from build123d import *

# Parameters (mm, degrees)
F0_W     = 2.8575
F0_H     = 5.08
F0_W_2   = 1.905
F0_W_3   = 5.3975
F0_H_2   = 5.128411484
F1_DEPTH = 4.445
F2_W     = 7.62
F2_H     = 83.82
F3_DEPTH = 5.3975
F4_W     = 17.018
F4_H     = 2.54
F4_W_2   = 2.45618
F4_W_3   = 14.56182
F5_DEPTH = 15.24
F6_DEPTH = 25.4


# Not quite as in the source:
# - a feature names something its author has since deleted; it is built from what else it names


with BuildPart() as f1:
    # F0 (on Front) → F1 (new body, symmetric)
    with BuildSketch(Plane.XZ):
        with Locations((-63.4578398415, 18.0266693214)):
            Rectangle(F0_W, F0_H)
        Polygon((-62.0290898415, 15.4866693214), (-64.8865898415, 15.4866693214), (-64.8865898415, 5.3266693214), (-1.3865898415, 5.3266693214), (-1.3865898415, 15.4866693214), (-6.7840898415, 15.4866693214), (-8.6890898415, 15.4866693214), (-10.5940898415, 15.4866693214), (-12.4990898415, 15.4866693214), (-13.314443469, 15.4866693214), (-14.4040898415, 15.4866693214), (-16.3090898415, 15.4866693214), (-18.2140898415, 15.4866693214), (-20.1190898415, 15.4866693214), (-22.0240898415, 15.4866693214), (-23.9290898415, 15.4866693214), (-25.8340898415, 15.4866693214), (-27.7390898415, 15.4866693214), (-29.6440898415, 15.4866693214), (-31.5490898415, 15.4866693214), (-33.4540898415, 15.4866693214), (-35.3590898415, 15.4866693214), (-37.2640898415, 15.4866693214), (-39.1690898415, 15.4866693214), (-41.0740898415, 15.4866693214), (-42.9790898415, 15.4866693214), (-44.8840898415, 15.4866693214), (-46.7890898415, 15.4866693214), (-48.6940898415, 15.4866693214), (-50.5990898415, 15.4866693214), (-52.5040898415, 15.4866693214), (-54.4090898415, 15.4866693214), (-56.3140898415, 15.4866693214), (-58.2190898415, 15.4866693214), (-60.1240898415, 15.4866693214), align=None)
        with Locations((-59.1715898415, 18.0266693214)):
            Rectangle(F0_W_2, F0_H)
        with Locations((-4.0853398415, 18.0266693214)):
            Rectangle(F0_W_3, F0_H)
        with Locations((-55.3615898415, 18.0266693214)):
            Rectangle(F0_W_2, F0_H)
        with Locations((-9.6415898415, 18.0266693214)):
            Rectangle(F0_W_2, F0_H)
        with Locations((-51.5515898415, 18.0266693214)):
            Rectangle(F0_W_2, F0_H)
        Polygon((-13.314443469, 15.4866693214), (-12.4990898415, 15.4866693214), (-12.4990898415, 20.5666693214), (-13.314443469, 20.5666693214), (-14.4040898415, 20.5666693214), (-14.4040898415, 15.4866693214), align=None)
        with Locations((-47.7415898415, 18.0266693214)):
            Rectangle(F0_W_2, F0_H)
        with Locations((-43.9315898415, 18.0266693214)):
            Rectangle(F0_W_2, F0_H)
        with Locations((-17.2615898415, 18.0266693214)):
            Rectangle(F0_W_2, F0_H)
        with Locations((-40.1215898415, 18.0266693214)):
            Rectangle(F0_W_2, F0_H)
        with Locations((-21.0715898415, 18.0266693214)):
            Rectangle(F0_W_2, F0_H)
        with Locations((-36.3115898415, 18.0508750634)):
            Rectangle(F0_W_2, F0_H_2)
        with Locations((-24.8815898415, 18.0266693214)):
            Rectangle(F0_W_2, F0_H)
        with Locations((-32.5015898415, 18.0266693214)):
            Rectangle(F0_W_2, F0_H)
        with Locations((-28.6915898415, 18.0266693214)):
            Rectangle(F0_W_2, F0_H)
    extrude(amount=F1_DEPTH, both=True)

    # F2 (on face) → F3 (join)
    with BuildSketch(Plane.YZ.offset(-1.3865898415)):
        Polygon((-4.445, 5.3266693214), (-4.445, 20.5666693214), (-43.815, 20.5666693214), (-43.815, 5.3266693214), (-37.465, 5.3266693214), (-29.845, 5.3266693214), align=None)
        with Locations((-33.655, -36.5833306786)):
            Rectangle(F2_W, F2_H)
    extrude(amount=-F3_DEPTH)

    # F4 (on face) → F5 (join)
    with BuildSketch(Plane.XY.offset(20.5666693214)):
        with Locations((-15.2930898415, -19.685)):
            Rectangle(F4_W, F4_H)
        with Locations((-22.5739998415, -42.545)):
            Rectangle(F4_W_2, F4_H)
        with Locations((-14.0649998415, -42.545)):
            Rectangle(F4_W_3, F4_H)
    extrude(amount=-F5_DEPTH)

    # F2 (on face) → F6 (join)
    with BuildSketch(Plane.YZ.offset(-1.3865898415)):
        Polygon((-19.840323447, -78.4933306786), (-29.845, -78.4933306786), (-37.465, -78.4933306786), (-47.469676553, -78.4933306786), (-47.469676553, -86.1133306786), (-19.840323447, -86.1133306786), align=None)
    extrude(amount=-F6_DEPTH)


solid = f1.part
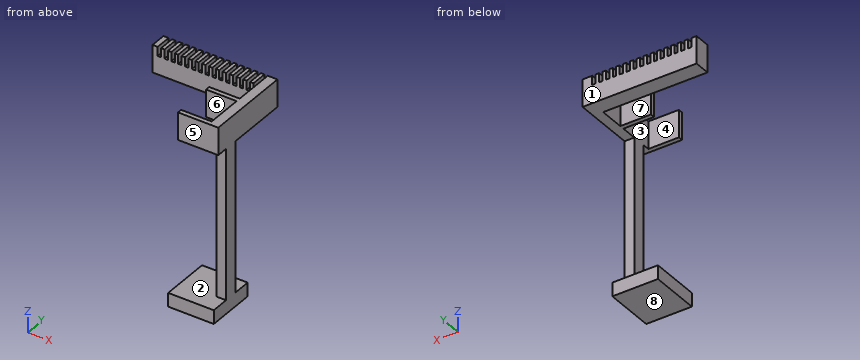
The listing builds one solid part. Answer for the finished solid, in the listing's coordinates (mm). Face numbers are marked on the shaded views. A direction names the side the tool comes from. Round coordinates to 2 decimals unless told otherwise and drop trailing zeros. Order: outer loops, then holes, each group sorted by start corner. A loop starts at its lowest first (then second) coordinate and runs counter-clockwise, first axis right, second up. Notation, with made-up numbers: (78.5, 10.25) - (103.5, 10.25) arc R33 cw to (103.5, 41.25) - close; hole circle Ø3 at (33, 73). An arc over 180 degrees is marked (long way). Write item = value, one per line. Start each with the question number.
1) Section C-C, the plane z = -23 is taken. Write down the section's boundary in (x, y) (3 decimals), plus the area to 3 significant figures.
2) Section B-B, the plane y = -6.5 is taken. Write down the section's boundary in (x, z).
3) Section A-A, the plane z = 6.5 is taken. Write down the section's boundary in (x, y) (3 decimals), plus the area to 3 significant figures.
4) For the marked faces 5, 6, 7 and 8, determine the directions among +Z, -Z, +X, -X, +Y, -Y from which every point of the face is accessible in a straight line to the end or side of a thin tool.
5) Given pin 1 (17 mm diameter, centred on x = -47.5, y = -11, fed in from -Z); pin 2 (2 mm diameter, centred on x = -23, y = -1.5, fed in from +Z); pin 3 (6.5 mm diameter, centred on x = -12, y = -29, fed in from +Z), each flat-ended and moving along its own axis, determine where each tip first touches the part or whether it passes through.
6) For a pull along Y with two mould halves and no side action, classify the marked faces 1, 2, 3 and 4 as released by +Y, released by -Y, zero draft, split by the parting line, or undercut.
7) Straight lines are drawn through the part: L1, parallel to Z at x = -14.5, y = -41.5; L2, parallel to Y at x = -45.5, z = 9 (3 decimals); L3, parallel to X at y = -31.5, z = -2. For each, find the intervals that lie inside material, in ascending order.
Results list:
q1.outline = (-6.784, -37.465) - (-1.387, -37.465) - (-1.387, -29.845) - (-6.784, -29.845) - close
q1.area = 41.1 mm^2
q2.outline = (-6.78, 5.33) - (-1.39, 5.33) - (-1.39, 20.57) - (-6.78, 20.57) - close
q3.outline = (-64.887, -4.445) - (-6.784, -4.445) - (-6.784, -18.415) - (-23.802, -18.415) - (-23.802, -20.955) - (-6.784, -20.955) - (-6.784, -41.275) - (-23.802, -41.275) - (-23.802, -43.815) - (-1.387, -43.815) - (-1.387, 4.445) - (-64.887, 4.445) - close
q3.area = 863 mm^2
q4.face_5 = +Z, +X, -X, -Y
q4.face_6 = +Z, -X
q4.face_7 = +Z, -Z, -X
q4.face_8 = -Z, +X, -X, +Y, -Y
q5.pin_1 = 5.33
q5.pin_2 = 20.57
q5.pin_3 = -78.49
q6.face_1 = released by +Y
q6.face_2 = zero draft
q6.face_3 = undercut
q6.face_4 = undercut
q7.L1 = -86.11 to -78.49, 5.33 to 20.57
q7.L2 = -4.445 to 4.445
q7.L3 = -6.78 to -1.39
